from build123d import *

# Parameters (mm, degrees)
SKETCH_3_R          = 1.5
CUT_EXTRUDE_4_DEPTH = 24.173260453
SKETCH_3_4_R        = 1.5
CUT_EXTRUDE_5_DEPTH = 24.173260453


with BuildPart() as part:
    # Sketch 2 → Revolve 1 (revolve)
    with BuildSketch(Plane(origin=(0, 0, 0), x_dir=(0, 0, -1), z_dir=(1, 0, 0)), mode=Mode.PRIVATE) as revolve_1_sk:
        Polygon((5, 0), (16, 0), (16, 5), (8, 5), (8, 8), (5, 8), align=None)
    revolve(revolve_1_sk.sketch.rotate(Axis((0, 18.095647444, 0), (0, -1, 0)), 180), axis=Axis((0, 18.095647444, 0), (0, -1, 0)))

    # Sketch 3 → Cut-Extrude 4 (cut, through all)
    with BuildSketch(Plane(origin=(0, 5, 0), x_dir=(1, 0, 0), z_dir=(0, 1, 0))):
        with Locations(Location((0, 12, 0), (0, 0, 270))):
            Circle(SKETCH_3_R)
    extrude(amount=-CUT_EXTRUDE_4_DEPTH, mode=Mode.SUBTRACT)

    # Sketch 3_4 → Cut-Extrude 5 (cut, through all)
    with BuildSketch(Plane(origin=(0, 5, 0), x_dir=(1, 0, 0), z_dir=(0, 1, 0))):
        with Locations(Location((0, -12, 0), (0, 0, 270))):
            Circle(SKETCH_3_4_R)
    extrude(amount=-CUT_EXTRUDE_5_DEPTH, mode=Mode.SUBTRACT)


solid = part.part
Here's how the part is built. I have some questions about the finished solid (model axes, mm). A direction names the side the tool comes from. Give positions to 0.01 mm unless a question says otherwise; leave off trailing zeros. Order: outer loops, then holes, each group sorted by start corner. A loop starts at its lowest first (then second) coordinate and runs counter-clockwise, first axis right, second up. Notation, with made-up numbers: M -20.75,16.5 L 20.25,16.5 A16 ccw 20.25,33.5 Z; hole C 24,28.5 d7. An arc over 180 degrees is marked long. Answer as a JSON object with one key per item and string values. Group by question number.
1) Suppose I cut it at B-B, the plane z = 0. Write out the boundary of the cut face in (x, y), plus the area to 3 significant figures.
2) We'd pull the mould along Z, two halves only. Please class faces 3 (the cylindrical face through (0.07, 2.54, 10.5)), 4 (the flat face through (5.2, 8, -0.1)), 5 (the cylindrical face through (7.81, 6.52, -1.73)), 6 (the cylindrical face through (0, 4, -5)): pulls with the +Z half, pulls with the -Z half, needs draft (parallel to the pull), parting line crosses it, or undercut.
3) I'm going to push flat-ended pins straight in: pin 1 Ø2 at (y, z) = (3.5, -2) entering from -X; pin 2 Ø5 at (x, z) = (0, -12) entering from +Y; pin 3 Ø1.5 at (x, y) = (9.5, 1) entering from +Z. Where does each tip first touch, or does it pass through?
4) Suppose I cut it at D-D, the plane y = 1.25. Write out the boundary of the cut face in (x, z).
5) Suppose I cut it at A-A, the plane x = 0. Write out the boundary of the cut face in (y, z).
6) Suppose I cut it at C-C, the plane x = -4. Write out the boundary of the cut face in (y, z), plus the area to 3 significant figures.
7) On a 3-axis mill with a long thin cutter (end or side, diameter ignored), from which of +Z, -Z, +X, -X, +Y, -Y can I reach the whole of each face in a straight line? I mean faces 1 (the flat face through (-7.3, 5, -3.8)), 2 (the cylindrical face through (0.07, 2.54, -13.5)). Say none if no direction works.
8) Please list where these lines run through material, in increasing order: L1, parallel to Y at x = 2.5, z = -9; L2, parallel to X at y = 6, z = 0; L3, parallel to X at y = 1, z = -13. Write a range as [from, to].
Results found:
{
 "1": {"outline": "M -16,0 L -5,0 L -5,8 L -8,8 L -8,5 L -16,5 Z; M 5,0 L 16,0 L 16,5 L 8,5 L 8,8 L 5,8 Z", "area": "128 mm²"},
 "2": {"face 3": "undercut", "face 4": "needs draft", "face 5": "parting line crosses it", "face 6": "undercut"},
 "3": {"pin 1": "x = -15.97", "pin 2": "y = 5", "pin 3": "z = 13.4"},
 "4": {"outline": "C 0,0 d32; hole C 0,0 d10; hole C 0,-12 d3; hole C 0,12 d3"},
 "5": {"outline": "M 0,-16 L 5,-16 L 5,-13.5 L 0,-13.5 Z; M 0,-10.5 L 5,-10.5 L 5,-8 L 8,-8 L 8,-5 L 0,-5 Z; M 0,5 L 8,5 L 8,8 L 5,8 L 5,10.5 L 0,10.5 Z; M 0,13.5 L 5,13.5 L 5,16 L 0,16 Z"},
 "6": {"outline": "M 0,-15.49 L 5,-15.49 L 5,-6.93 L 8,-6.93 L 8,-3 L 0,-3 Z; M 0,3 L 8,3 L 8,6.93 L 5,6.93 L 5,15.49 L 0,15.49 Z", "area": "148 mm²"},
 "7": {"face 1": "+Y", "face 2": "+Y, -Y"},
 "8": {"L1": "[0, 5]", "L2": "[-8, -5], [5, 8]", "L3": "[-9.33, -1.12], [1.12, 9.33]"}
}
